For this review, use the dimensioned drawing (mm, ordinates from the lowest corner) and the shaded views. A direction names the side the tool comes from. Coordinates: 2 decimals unless noted, no trailing zeros. Write each loop counter-clockwise with the first axis right and the second up, starting at its lowest first coordinate (ties: lowest second). Pieces come first, ordered by that corner, then holes. Notation, with made-up numbers: (11.25, 64.25) - (60.25, 64.25) arc R16 cw to (60.25, 87.25) - close; hole circle Ø7 at (34, 8). An arc over 180 degrees is marked (long way). Use one line per item in the form item = value. Start each with the question number.
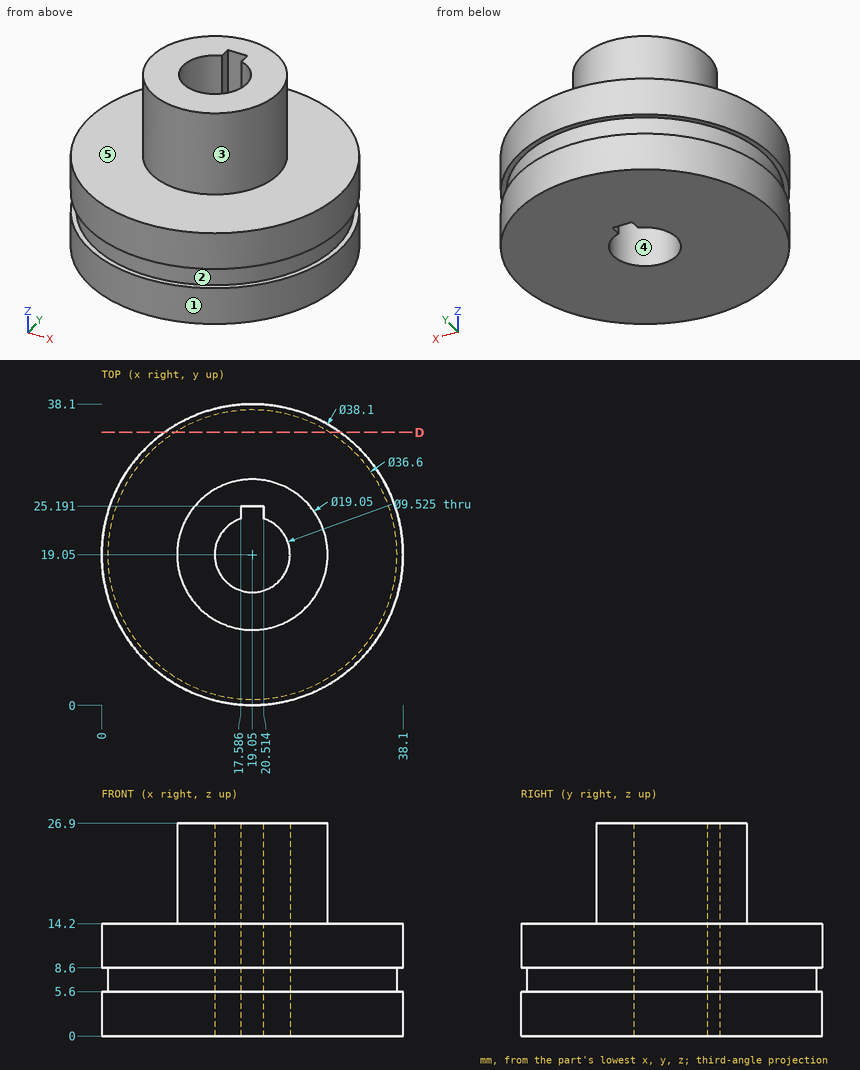
1. For the marked faces 1 and 2, list the 3-axis set-ups (+Z, -Z, +X, -X, +Y, -Y) from which the entire face can be reached by the end or side of a thin tool; tool diameter is ignored.
2. The part is to be moulded in two halves that separate along X. For the marked faces 3, 4 and 5, say which applies: released by +X, released by -X, zero draft, split by the parting line, or undercut.
3. Take a section at D-D (y = 34.5). State the section outline as (x, z) points (1 decimal).
4. For P1, Ø1, axis at y = 19.5, z = 20, coming from the +X side (3 decimals); P2, Ø10, axis at y = 13.5, z = 23.5, coming from the -X side; P3, Ø3, axis at x = 12, y = 22.5, coming from the -Z side; P4, Ø3, axis at x = 19, z = 7.5, coming from the -Y side, all flat-tipped, find the tip position at first contact; note any pin that passes through.
5. For L1, parallel to Y at x = 19.05, z = 20.5 (1 decimal); L2, parallel to Y at x = 19.05, z = 13.25; L3, parallel to Z at x = 12, y = 34, list the stretches that pass through material, from the lowest coordinate up.
Returned:
q1.face_1 = +Z, -Z
q1.face_2 = none
q2.face_3 = split by the parting line
q2.face_4 = undercut
q2.face_5 = zero draft
q3.outline = (7.9, 0) - (30.2, 0) - (30.2, 5.6) - (28.9, 5.6) - (28.9, 8.6) - (30.2, 8.6) - (30.2, 14.2) - (7.9, 14.2) - (7.9, 8.6) - (9.2, 8.6) - (9.2, 5.6) - (7.9, 5.6) - close
q4.P1 = 28.575
q4.P2 = 9.54
q4.P3 = 0
q4.P4 = 0
q5.L1 = 9.5 to 14.3, 25.2 to 28.6
q5.L2 = 0 to 14.29, 25.19 to 38.1
q5.L3 = 0 to 14.2
